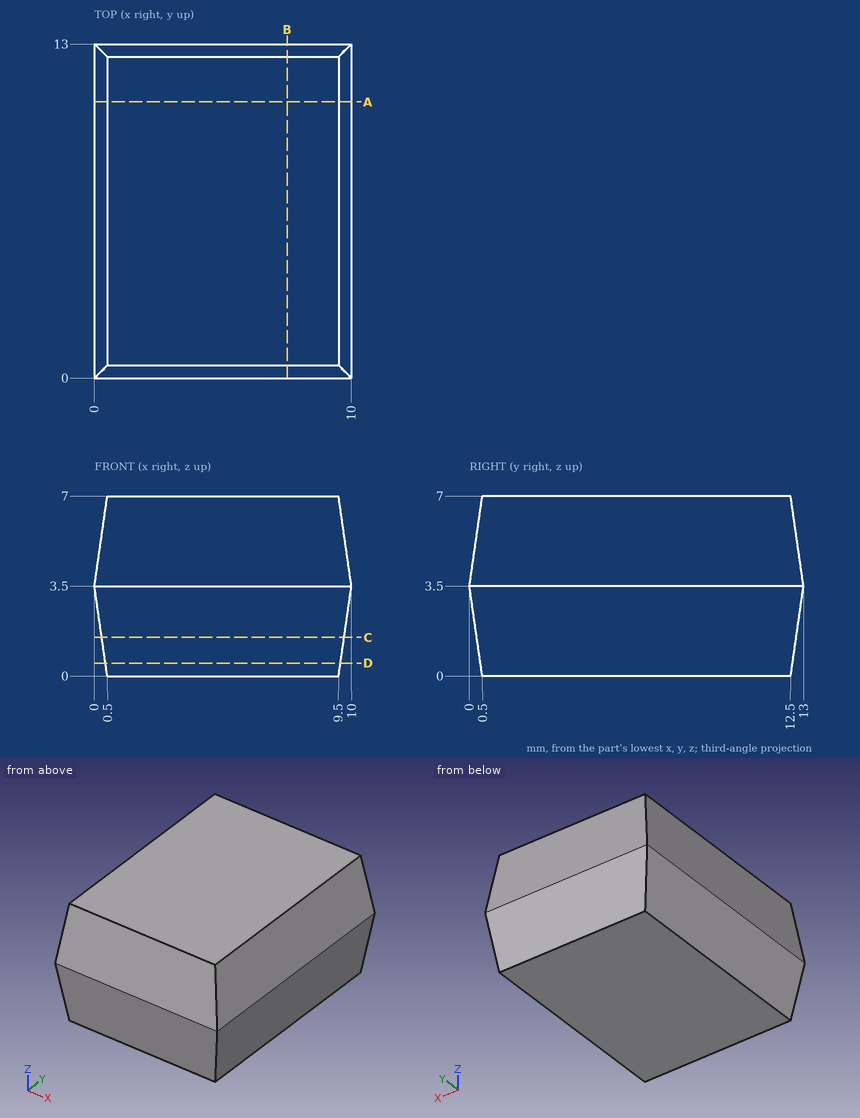
Verification items for this drawing (mm, ordinates from the low corner). Give positions to 0.01 mm unless a question says otherwise; leave off trailing zeros. Write each loop counter-clockwise with the first axis right and the second up, starting at its lowest first coordinate (ties: lowest second). Pieces come first, ordered by that corner, then holes.
1) Section check D-D, the plane z = 0.5. Record the boundary of the cut face in (x, y), and give its area (3 significant figures).
2) Section check B-B, the plane x = 7.5. Record the boundary of the cut face in (y, z), and give its area (3 significant figures).
3) Section check A-A, the plane y = 10.75. Record the boundary of the cut face in (x, z), and give its area (3 significant figures).
4) Material ranges on L1, parallel to Y at x = 1, z = 5; L2, parallel to Y at x = 2.5, z = 5.75; L3, parallel to X at y = 3.25, z = 1.5, recorded low to high.
5) Section check C-C, the plane z = 1.5. Record the boundary of the cut face in (x, y).
6) Gauge pin test, flat ends, axial feed: pin 1 (1 mm diameter, centred on y = 9, z = 1, fed in from +X); pin 2 (4 mm diameter, centred on x = 8, z = 4, fed in from -Y); pin 3 (3 mm diameter, centred on x = 4, z = 1, fed in from -Y). Record the tip position at first contact, or that the pin passes through.
Computed:
1. outline: (0.43, 0.43) - (9.57, 0.43) - (9.57, 12.57) - (0.43, 12.57) - close
1. area: 111 mm2
2. outline: (0, 3.5) - (0.5, 0) - (12.5, 0) - (13, 3.5) - (12.5, 7) - (0.5, 7) - close
2. area: 87.5 mm2
3. outline: (0, 3.5) - (0.5, 0) - (9.5, 0) - (10, 3.5) - (9.5, 7) - (0.5, 7) - close
3. area: 66.5 mm2
4. L1: y = 0.21 to 12.79
4. L2: y = 0.32 to 12.68
4. L3: x = 0.29 to 9.71
5. outline: (0.29, 0.29) - (9.71, 0.29) - (9.71, 12.71) - (0.29, 12.71) - close
6. pin 1: stops at x = 9.71
6. pin 2: stops at y = 0
6. pin 3: stops at y = 0.14
